Read the model definition and answer for the solid it produces. Units are mm, in the model's axes. A direction names the side the tool comes from. Coordinates: 2 decimals unless noted, no trailing zeros. Loops run counter-clockwise (first coordinate to the right, second up) from the corner with the lowest first, then second, coordinate; pieces in that order, holes last. Notation, with made-up numbers: (-11.5, 13) -> (-4.5, 13) arc R29 cw to (-4.5, 45) -> close; hole circle Ø10 at (66.5, -14.75). An arc over 180 degrees is marked (long way). Answer as CSV lines item,"result".
```python
from build123d import *

# Parameters (mm, degrees)
F0_W     = 57.15
F0_H     = 45.72
F0_R     = 3.175
F1_DEPTH = 6.096
F2_R     = 4.572
F3_DEPTH = 45.721
F4_R     = 4.7625
F5_DEPTH = 12.7
F6_R     = 4.7625
F7_DEPTH = 12.7


with BuildPart() as f1:
    # F0 (on Front) → F1 (new body, symmetric)
    with BuildSketch(Plane.XZ):
        with Locations((0, 0.635)):
            Rectangle(F0_W, F0_H)
        with BuildLine():
            ThreePointArc((-3.302, -4.826), (-8.128, 0), (-3.302, 4.826))
            Line((-3.302, 4.826), (18.288, 4.826))
            ThreePointArc((18.288, 4.826), (23.114, 0), (18.288, -4.826))
            Line((18.288, -4.826), (-3.302, -4.826))
        make_face(mode=Mode.SUBTRACT)
        with Locations((-12.7, 15.875)):
            Circle(F0_R, mode=Mode.SUBTRACT)
        with Locations((12.7, 15.875)):
            Circle(F0_R, mode=Mode.SUBTRACT)
    extrude(amount=F1_DEPTH, both=True)

    # F2 (on face) → F3 (cut, through all)
    with BuildSketch(Plane.XY.offset(23.495)):
        with Locations((-22.225, 0)):
            Circle(F2_R)
        with Locations((22.225, 0)):
            Circle(F2_R)
    extrude(amount=-F3_DEPTH, mode=Mode.SUBTRACT)

    # F4 (on face) → F5 (cut)
    with BuildSketch(Plane.XY.offset(23.495)):
        with Locations((-22.225, 0)):
            Circle(F4_R)
        with Locations((22.225, 0)):
            Circle(F4_R)
    extrude(amount=-F5_DEPTH, mode=Mode.SUBTRACT)

    # F6 (on face) → F7 (cut)
    with BuildSketch(Plane(origin=(0, 0, -22.225), x_dir=(1, 0, 0), z_dir=(0, 0, -1))):
        with Locations((22.225, 0)):
            Circle(F6_R)
        with Locations((-22.225, 0)):
            Circle(F6_R)
    extrude(amount=-F7_DEPTH, mode=Mode.SUBTRACT)


solid = f1.part
```
Q1. A cutting plane is placed at A-A, the plane y = 0. Give the number of separate pieces and of enclosed holes in the cut face, and give its area (3 significant figures).
Results:
separate pieces,"3"
enclosed holes,"2"
area,"1,460 mm²"
Q2. Given pin 1 Ø12 at (x, z) = (7, 2.5) entering from +Y, flat-ended and moving along its own axis, determine where the tip first touches the part or whether it passes through.
Results:
pin 1,"stops at y = 6.1"
Q3. A cutting plane is placed at D-D, the plane x = 21. Write down the section's boundary in (y, z) (3 decimals).
Results:
outline,"(-6.096, -22.225) -> (-4.602, -22.225) -> (-4.602, -9.525) -> (-4.405, -9.525) -> (-4.405, -3.992) -> (-6.096, -3.992) -> close; (-6.096, 3.992) -> (-4.405, 3.992) -> (-4.405, 10.795) -> (-4.602, 10.795) -> (-4.602, 23.495) -> (-6.096, 23.495) -> close; (4.405, -9.525) -> (4.602, -9.525) -> (4.602, -22.225) -> (6.096, -22.225) -> (6.096, -3.992) -> (4.405, -3.992) -> close; (4.405, 3.992) -> (6.096, 3.992) -> (6.096, 23.495) -> (4.602, 23.495) -> (4.602, 10.795) -> (4.405, 10.795) -> close"
Q4. Find the intervals of material crossed by probe 1 along X at (y, z) = (-0.25, 11) (3 decimals); probe 2 along Z at (x, y) = (1.5, -0.75) (3 decimals); probe 3 along X at (y, z) = (1, 1) (3 decimals), in increasing order. Write a range as [from, to].
Results:
probe 1,"x = [-28.575, -26.981], [-17.469, 17.469], [26.981, 28.575]"
probe 2,"z = [-22.225, -4.826], [4.826, 23.495]"
probe 3,"x = [-28.575, -26.686], [-17.764, -8.023], [26.686, 28.575]"
Q5. For a pull along Y with two mould halves and no side action, classify faces 1 (the face through (26.586, 1.373, 0.777)), 2 (the face through (-8.127, -0.085, -0.106)), 3 (the face through (0, -6.096, 6)) as pulls with the +Y half, pulls with the -Y half, needs draft (parallel to the pull), parting line crosses it, or undercut.
Results:
face 1,"undercut"
face 2,"needs draft"
face 3,"pulls with the -Y half"
Q6. A cutting plane is placed at B-B, the plane x = -12.7. Write down the section's boundary in (y, z) (3 decimals).
Results:
outline,"(-6.096, -22.225) -> (6.096, -22.225) -> (6.096, 12.7) -> (-6.096, 12.7) -> close; (-6.096, 19.05) -> (6.096, 19.05) -> (6.096, 23.495) -> (-6.096, 23.495) -> close"
Q7. For faces 4 (the face through (-17.682, -1.431, -15.964)), 5 (the face through (17.467, 0.209, 17.234)), 6 (the face through (23.113, 5.022, 0.106)), determine the directions among +Z, -Z, +X, -X, +Y, -Y from which every point of the face is accessible in a straight line to the end or side of a thin tool.
Results:
face 4,"-Z"
face 5,"+Z"
face 6,"+Y, -Y"
Q8. A cutting plane is placed at C-C, the plane z = 4. Write down the section's boundary in (x, y) (1 decimal).
Results:
outline,"(-28.6, -6.1) -> (-6, -6.1) -> (-6, 6.1) -> (-28.6, 6.1) -> close; (21, -6.1) -> (28.6, -6.1) -> (28.6, 6.1) -> (21, 6.1) -> (21, 4.4) arc R4.6 cw (long way) to (21, -4.4) -> close; hole circle Ø9.1 at (-22.2, 0)"
